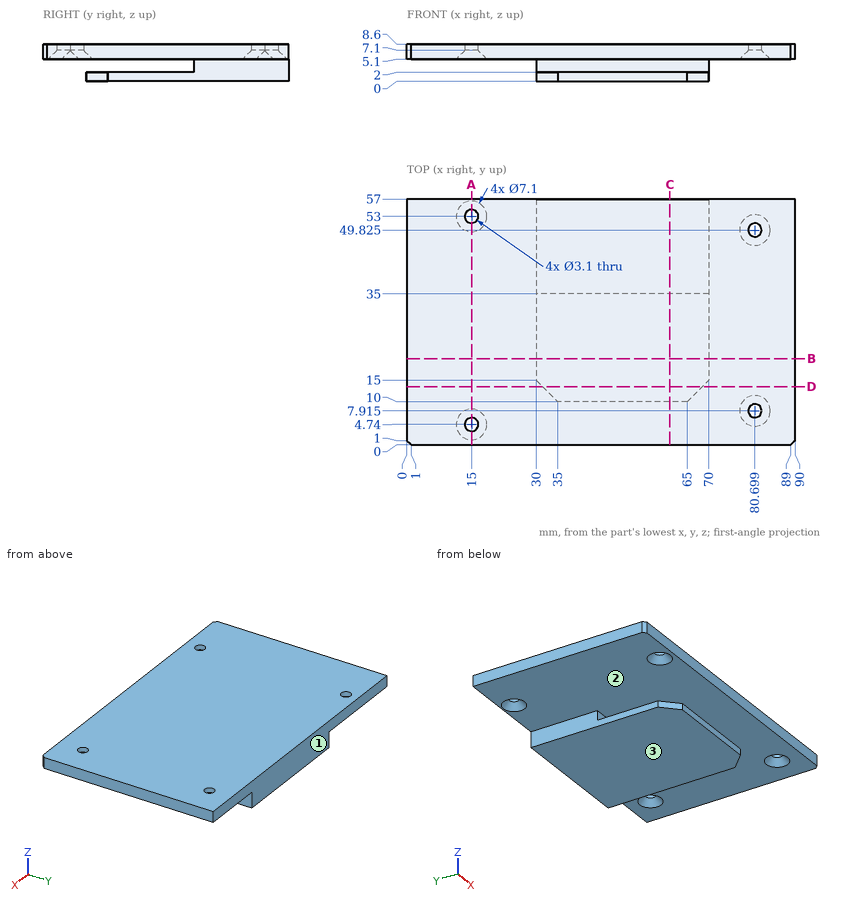
Input: dimensioned drawing with shaded views. Units: mm. Origin: part minimum x, y, z. Round coordinates to 2 decimals unless told otherwise and drop trailing zeros. Order: outer loops, then holes, each group sorted by start corner. A loop starts at its lowest first (then second) coordinate and runs counter-clockwise, first axis right, second up. Notation, with made-up numbers: (89, 0) - (132, 0) arc R20 ccw to (132, 24) - close; hole circle Ø7 at (-16.5, 54). An arc over 180 degrees is marked (long way). Answer as a JSON object with one key per item and string values. Group by question number.
(1) Cut plane A-A (x = 15). Return loops of the section in (y, z).
(2) Pin query (flat end, axial travel): P1, Ø3, axis at x = 80.699, y = 7.915, coming from the -Z side; P2, Ø1.5, axis at y = 34.5, z = 3.5, coming from the -X side; P3, Ø1.5, axis at y = 44.5, z = 2, coming from the +X side; P4, Ø4, axis at x = 42.5, z = 1, coming from the -Y side. Return the tip coordinate at first contact, or that it passes through.
(3) Draft query along Z for the marked faces 1, 2 and 3. Return one class per face: released by +Z, released by -Z, zero draft, split by the parting line, or undercut.
(4) Cut plane D-D (y = 13.5). Return loops of the section in (x, z), then the cut area to 3 significant figures.
(5) Material intervals for probe 1 along Y at (x, z) = (15, 7.5); probe 2 along Z at (x, y) = (39, 14); probe 3 along Z at (x, y) = (27, 45), sorted ascending. Write a range as from..to.
(6) Cut plane B-B (y = 20). Return loops of the section in (x, z), then the cut area to 3 significant figures.
(7) Cut plane C-C (x = 61). Return loops of the section in (y, z), then the cut area to 3 significant figures.
Here are the results:
{
 "1": {"outline": "(0, 5.1) - (1.19, 5.1) - (3.19, 7.1) - (3.19, 8.6) - (0, 8.6) - close; (6.29, 7.1) - (8.29, 5.1) - (49.45, 5.1) - (51.45, 7.1) - (51.45, 8.6) - (6.29, 8.6) - close; (54.55, 7.1) - (56.55, 5.1) - (57, 5.1) - (57, 8.6) - (54.55, 8.6) - close"},
 "2": {"P1": "passes through", "P2": "stops at x = 30", "P3": "stops at x = 70", "P4": "stops at y = 10"},
 "3": {"face 1": "zero draft", "face 2": "undercut", "face 3": "released by -Z"},
 "4": {"outline": "(0, 5.1) - (90, 5.1) - (90, 8.6) - (0, 8.6) - close; (31.5, 0) - (68.5, 0) - (68.5, 2) - (31.5, 2) - close", "area": "389 mm^2"},
 "5": {"probe 1": "y = 0..3.19, 6.29..51.45, 54.55..57", "probe 2": "z = 0..2, 5.1..8.6", "probe 3": "z = 5.1..8.6"},
 "6": {"outline": "(0, 5.1) - (90, 5.1) - (90, 8.6) - (0, 8.6) - close; (30, 0) - (70, 0) - (70, 2) - (30, 2) - close", "area": "395 mm^2"},
 "7": {"outline": "(0, 5.1) - (35, 5.1) - (35, 2) - (10, 2) - (10, 0) - (57, 0) - (57, 8.6) - (0, 8.6) - close", "area": "362 mm^2"}
}
